from build123d import *

# Parameters (mm, degrees)
SKETCH1_W           = 75
SKETCH1_H           = 40
BOSS_EXTRUDE1_DEPTH = 40
SKETCH2_R           = 10.5
CUT_EXTRUDE1_DEPTH  = 30
SKETCH3_R           = 1.55
CUT_EXTRUDE2_DEPTH  = 40
FILLET1_R           = 2.5
SKETCH6_R           = 10.5
SKETCH4_R           = 10.5


with BuildPart() as part:
    # Sketch1 → Boss-Extrude1 (new body)
    with BuildSketch(Plane(origin=(0, 0, 0), x_dir=(1, 0, 0), z_dir=(0, 1, 0))):
        Rectangle(SKETCH1_W, SKETCH1_H)
    extrude(amount=BOSS_EXTRUDE1_DEPTH)

    # Sketch2 → Cut-Extrude1 (cut)
    with BuildSketch(Plane.ZY.offset(37.5)):
        with Locations((0, 17.5)):
            Circle(SKETCH2_R)
    extrude(amount=-CUT_EXTRUDE1_DEPTH, mode=Mode.SUBTRACT)

    # Sketch3 → Cut-Extrude2 (cut)
    with BuildSketch(Plane(origin=(0, 40, 0), x_dir=(1, 0, 0), z_dir=(0, 1, 0))):
        with Locations((-25, 15.25)):
            Circle(SKETCH3_R)
        with Locations((25, 15.25)):
            Circle(SKETCH3_R)
        with Locations((-25, -15.25)):
            Circle(SKETCH3_R)
        with Locations((25, -15.25)):
            Circle(SKETCH3_R)
    extrude(amount=-CUT_EXTRUDE2_DEPTH, mode=Mode.SUBTRACT)

    # Fillet1
    fillet1_edges = [part.edges().sort_by_distance(p)[0] for p in [
        (-37.5, 40, 0),
        (-37.5, 17.5, -10.5),
        (0, 40, 20),
        (37.5, 40, 0),
        (0, 0, 20),
        (-37.5, 0, 0),
        (0, 0, -20),
        (37.5, 0, 0),
        (37.5, 20, 20),
        (-37.5, 20, 20),
        (-37.5, 20, -20),
        (37.5, 20, -20),
        (0, 40, -20),
    ]]
    fillet(fillet1_edges, radius=FILLET1_R)

    # Sketch6 → Cut-Loft1 section 0
    with BuildSketch(Plane(origin=(0, 0, 0), x_dir=(1, 0, 0), z_dir=(0, 1, 0))):
        with Locations((-20, 0)):
            Circle(SKETCH6_R)
    # Sketch4 → Cut-Loft1 section 1
    with BuildSketch(Plane(origin=(0, 40, 0), x_dir=(1, 0, 0), z_dir=(0, 1, 0))):
        with Locations((20, 0)):
            Circle(SKETCH4_R)
    loft(mode=Mode.SUBTRACT)


solid = part.part
Part model, mm, in its own coordinate system. A direction names the side the tool comes from. Give positions to 0.01 mm unless a question says otherwise; leave off trailing zeros. Order: outer loops, then holes, each group sorted by start corner. A loop starts at its lowest first (then second) coordinate and runs counter-clockwise, first axis right, second up. Notation, with made-up numbers: (-30.5, 43) - (-4.5, 43) arc R19 cw to (-4.5, 48) - close; hole circle Ø8 at (-14.75, 34.5). An arc over 180 degrees is marked (long way). Use a Markdown table: item, result.
1) Two-plate mould, pull along Z, no slides. Class faces 1 (the cylindrical face through (37, 20, -19)), 2 (the cylindrical face through (-37, 1, 0)), 3 (the cylindrical face through (-25.202, 20.28, -16.787)): +Z half, -Z half, draft (parallel to the pull), parting line (faces both ways), or undercut.
Checked values:
| item | result |
|---|---|
| face 1 | -Z half |
| face 2 | draft |
| face 3 | undercut |
2) Flat gauge pins, fed straight in: P1, Ø4, axis at y = 21, z = 3.5, coming from the -X side; P2, Ø6, axis at y = 15.5, z = 7.5, coming from the -X side. Where does each tip first touch, or does it go through?
Checked values:
| item | result |
|---|---|
| P1 | x = -7.5 |
| P2 | x = -36.11 |
3) Probe L1, parallel to X at y = 22, z = 15.25; L2, parallel to Z at x = 25, y = 27; L3, parallel to Z at x = -25, y = 19. List the from-to ranges inside material, lowest first. Write a range as from..to.
Checked values:
| item | result |
|---|---|
| L1 | -37.5..-26.55, -23.45..23.45, 26.55..37.5 |
| L2 | -20..-16.8, -13.7..13.7, 16.8..20 |
| L3 | -20..-16.8, -13.7..-10.39, 10.39..13.7, 16.8..20 |
4) 3-axis set-ups, long thin cutter, end or side, ignore diameter. For faces 4 (the flat face through (-7.5, 24, 0)), 5 (the cylindrical face through (37, 20, 19)): which of +Z, -Z, +X, -X, +Y, -Y reach the whole face in a straight line?
Checked values:
| item | result |
|---|---|
| face 4 | -X |
| face 5 | +Z, +X, +Y, -Y |
5) Saw through at A-A on z = 15.25. List the corners of the cut face in (x, y).
Checked values:
| item | result |
|---|---|
| outline | (-37.5, 2.5) arc R2.5 ccw to (-35, 0) - (-26.55, 0) - (-26.55, 40) - (-35, 40) arc R2.5 ccw to (-37.5, 37.5) - close; (-23.45, 0) - (23.45, 0) - (23.45, 40) - (-23.45, 40) - close; (26.55, 0) - (35, 0) arc R2.5 ccw to (37.5, 2.5) - (37.5, 37.5) arc R2.5 ccw to (35, 40) - (26.55, 40) - close |
6) Saw through at B-B on x = -25. Count the separate pieces of the cut face and the enclosed holes in it, plus the area to 3 significant figures.
Checked values:
| item | result |
|---|---|
| separate pieces | 3 |
| enclosed holes | 1 |
| area | 928 mm² |
